Check sheet for the modelled part. Datum: model origin and axes. Units: mm. Face numbers are marked on the shaded views. A direction names the side the tool comes from. Give positions to 0.01 mm unless a question says otherwise; leave off trailing zeros. Order: outer loops, then holes, each group sorted by start corner. A loop starts at its lowest first (then second) coordinate and runs counter-clockwise, first axis right, second up. Notation, with made-up numbers: (37.5, 57.25) - (84.5, 57.25) arc R18 ccw to (84.5, 85.25) - close; hole circle Ø6 at (58.5, -12). An arc over 180 degrees is marked (long way). Answer in a Markdown table with one row per item.
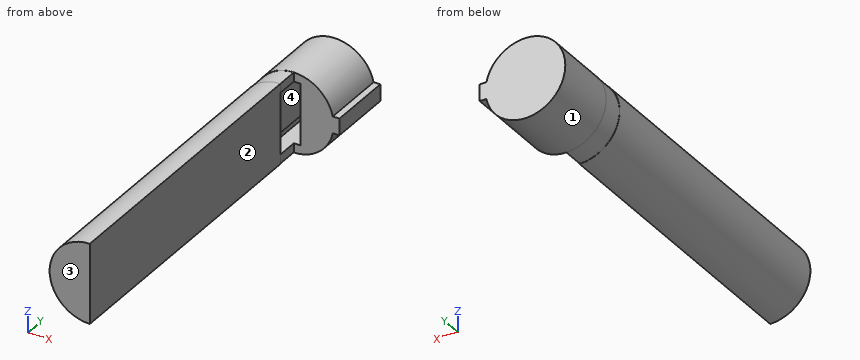
from build123d import *

# Parameters (mm, degrees)
PAD_DEPTH    = 15
POCKET_DEPTH = 13
PAD001_DEPTH = 5
PAD002_DEPTH = 70


with BuildPart() as part:
    # Sketch → Pad (new body)
    with BuildSketch(Plane.XZ):
        with BuildLine():
            ThreePointArc((8.889624, 1.945402), (-9.099882, -0.046426), (8.90901, -1.854598))
            Line((10.40901, -1.854598), (8.90901, -1.854598))
            Line((10.40901, 1.945402), (10.40901, -1.854598))
            Line((8.889624, 1.945402), (10.40901, 1.945402))
        make_face()
    extrude(amount=PAD_DEPTH)

    # Sketch001 (on Face6 of Pad) → Pocket (cut)
    with BuildSketch(Plane.XZ.offset(15)):
        Polygon((-1.5, 7), (1.5, 7), (1.5, -7), (-3.348355, -7), (-3.348355, -3.808815), (-1.5, -3.808815), align=None)
    extrude(amount=-POCKET_DEPTH, mode=Mode.SUBTRACT)

    # Sketch002 (on Face5 of Pocket) → Pad001 (join)
    with BuildSketch(Plane.XZ.offset(15)):
        with BuildLine():
            Line((0, 7), (-1.5, 7))
            Line((-1.5, 7), (-1.5, -3.808815))
            Line((-1.5, -3.808815), (-3.348355, -3.808815))
            Line((-3.348355, -3.808815), (-3.348355, -7))
            Line((-3.348355, -7), (0, -7))
            Line((0, -7), (0, -9.054887))
            ThreePointArc((0, 9.054887), (-9.054887, 0), (0, -9.054887))
            Line((0, 7), (0, 9.054887))
        make_face()
    extrude(amount=PAD001_DEPTH)

    # Sketch003 (on Face14 of Pad001) → Pad002 (join)
    with BuildSketch(Plane.XZ.offset(20)):
        with BuildLine():
            ThreePointArc((0.053764, 9.099841), (-9.1, 0), (0.053764, -9.099841))
            Line((0.053764, 9.099841), (0.053764, -9.099841))
        make_face()
    extrude(amount=PAD002_DEPTH)


solid = part.part
(1) Access from +Z, -Z, +X, -X, +Y, -Y to the whole of each face (thin tool, end or side, straight path). Record for the marked faces 1 and 2.
Geometry says:
| item | result |
|---|---|
| face 1 | +Y, -Y |
| face 2 | +Z, -Z, +X, -Y |
(2) Cross-section at A-A, the plane z = 0. Record the cut outline in (x, y), then the cut area to 3 significant figures.
Geometry says:
| item | result |
|---|---|
| outline | (-9.1, -90) - (0.05, -90) - (0.05, -20) - (-1.5, -20) - (-1.5, -2) - (1.5, -2) - (1.5, -15) - (10.41, -15) - (10.41, 0) - (-9.1, 0) - (-9.1, -15) - (-9.05, -15) - (-9.05, -20) - (-9.1, -20) - close |
| area | 932 mm² |
(3) Thickness scan on L1, parallel to Y at x = -0.25, z = -3.5; L2, parallel to Y at x = 7.25, z = 0.75; L3, parallel to X at y = -63, z = 0.5. Record the ranges inside material, lowest first.
Geometry says:
| item | result |
|---|---|
| L1 | -90 to -20, -2 to 0 |
| L2 | -15 to 0 |
| L3 | -9.09 to 0.05 |
(4) Cross-section at D-D, the plane z = -4.75. Record the cut outline in (x, y).
Geometry says:
| item | result |
|---|---|
| outline | (-7.76, -90) - (0.05, -90) - (0.05, -20) - (-3.35, -20) - (-3.35, -2) - (1.5, -2) - (1.5, -15) - (7.76, -15) - (7.76, 0) - (-7.76, 0) - (-7.76, -15) - (-7.71, -15) - (-7.71, -20) - (-7.76, -20) - close |
(5) Cross-section at B-B, the plane x = -4.25. Record the cut outline in (y, z).
Geometry says:
| item | result |
|---|---|
| outline | (-90, -8.05) - (-20, -8.05) - (-20, -8) - (-15, -8) - (-15, -8.05) - (0, -8.05) - (0, 8.05) - (-15, 8.05) - (-15, 8) - (-20, 8) - (-20, 8.05) - (-90, 8.05) - close |
(6) Mould release check, pull along Y, two halves, no side actions. Record for the marked faces 3 and 4: pulls with the +Y half, pulls with the -Y half, needs draft (parallel to the pull), parting line crosses it, or undercut.
Geometry says:
| item | result |
|---|---|
| face 3 | pulls with the -Y half |
| face 4 | undercut |
(7) Gauge pin test, flat ends, axial feed: P1, Ø9, axis at y = -42.5, z = -0.5, coming from the +X side; P2, Ø1.6, axis at y = -15.5, z = -5.5, coming from the +X side; P3, Ø8, axis at x = 7, y = -52.5, coming from the +Z side; P4, Ø1, axis at y = -16.5, z = 8, coming from the +X side. Record the tip position at first contact, or that the pin passes through.
Geometry says:
| item | result |
|---|---|
| P1 | x = 0.05 |
| P2 | x = 7.68 |
| P3 | through |
| P4 | x = 0 |
